For this review, take the finished solid that the model builds, in its own axes (mm). A direction names the side the tool comes from. Round coordinates to 2 decimals unless told otherwise and drop trailing zeros. Loops run counter-clockwise (first coordinate to the right, second up) from the corner with the lowest first, then second, coordinate; pieces in that order, holes last. Notation, with made-up numbers: M 56,70 L 103,70 A30 ccw 103,102 Z; hole C 65.25,-30 d6. An arc over 180 degrees is marked long. One line per question, with ' | ' between items. Start each with the question number.
1) We need section A-A (x = -64). Give the boundary of the cut face in (y, z), and give its area (3 significant figures).
2) We need section D-D (z = 4.5). Give the boundary of the cut face in (x, y), and give its area (3 significant figures).
3) We need section B-B (z = 48). Give the boundary of the cut face in (x, y), and give its area (3 significant figures).
4) We need section C-C (y = 21). Give the boundary of the cut face in (x, z).
5) For pin 1 Ø12 at (x, y) = (-50.5, 51.5) entering from +Z; pin 2 Ø9 at (x, y) = (72.5, 54.5) entering from -Z; pin 3 Ø10 at (x, z) = (69, 23) entering from -Y; pin 4 Ø11 at (y, z) = (-12, 52.5) entering from +X, all flat-tipped, find the tip position at first contact; note any pin that passes through.
6) For probe 1 along X at (y, z) = (66.5, 5); probe 2 along Z at (x, y) = (64, 56); probe 3 along Y at (x, z) = (-70.5, 34), list the stretches that pass through material, from the lowest coordinate up. Write a range as from..to.
7) For faces 1 (the face through (5, -10, 50)), 2 (the face through (70, 57, 52.5)), 3 (the face through (-60, 40, 27)), 4 (the face through (-70, 62.5, 27)), 5 (the face through (0, -10, 45)), list the 3-axis set-ups (+Z, -Z, +X, -X, +Y, -Y) from which the entire face can be reached by the end or side of a thin tool; tool diameter is ignored.
8) Mouldability with a two-part tool opening along X and no side actions: class faces 6 (the face through (60, 32, 27)), 7 (the face through (-5, -10, 50)), 8 (the face through (1, -5, 27)) as pulls with the +X half, pulls with the -X half, needs draft (parallel to the pull), parting line crosses it, or undercut.
Autodesk Inventor part; units mm, degrees
ref_plane "YZ Plane" through (0, 0, 0) normal (1, 0, 0) x (0, 1, 0)
ref_plane "XZ Plane" through (0, 0, 0) normal (0, 1, 0) x (-1, 0, 0)
ref_plane "XY Plane" through (0, 0, 0) normal (0, 0, 1) x (1, 0, 0)
sketch "Boceto1" plane through (0, 0, 0) normal (0, 0, 1) x (1, 0, 0)
  line L0 (-80, 5) -> (80, 5)
  line L1 (80, 5) -> (80, -5)
  line L2 (80, -5) -> (-80, -5)
  line L3 (-80, -5) -> (-80, 5)
  line L4 (-80, 5) -> (80, -5) construction
  line L5 (80, 5) -> (-80, -5) construction
  point P0 (0, 0)
  dimension "d0" = 160
  dimension "d1" = 10
extrude "Extrusión1" add sketch "Boceto1" along normal blind 55
sketch "Boceto2" plane through (-80, 5, 0) normal (0, 1, 0) x (1, 0, 0)
  line L0 (0, 0) -> (0, -55)
  line L1 (0, -55) -> (160, -55)
  line L2 (0, 0) -> (20, 0)
  line L3 (20, 0) -> (20, -55)
  line L4 (20, -55) -> (0, -55)
  line L5 (0, -55) -> (0, 0)
  line L6 (160, 0) -> (160, -55)
  line L7 (160, 0) -> (140, 0)
  line L8 (140, 0) -> (140, -55)
  line L9 (140, -55) -> (160, -55)
  line L10 (160, -55) -> (160, 0)
  point P0 (80, 0)
  dimension "d4" = 20
  dimension "d5" = 20
extrude "Extrusión2" add sketch "Boceto2" along normal blind 70
sketch "Boceto3" plane through (-80, -5, 0) normal (-1, 0, 0) x (0, 0, 1)
  line L0 (0, 80) -> (55, 80)
  line L1 (20.5, 67.5) -> (34.5, 67.5)
  line L2 (34.5, 67.5) -> (34.5, 53.5)
  line L3 (34.5, 53.5) -> (20.5, 53.5)
  line L4 (20.5, 53.5) -> (20.5, 67.5)
  line L5 (20.5, 67.5) -> (34.5, 53.5) construction
  line L6 (34.5, 67.5) -> (20.5, 53.5) construction
  line L7 (0, 0) -> (0, 80)
  point P0 (0, 5)
  point P1 (27.5, 60.5)
  dimension "d10" = 14
  dimension "d11" = 14
  dimension "d12" = 20.5
  dimension "d13" = 12.5
extrude "Extrusión3" cut sketch "Boceto3" against normal blind 70
sketch "Boceto4" plane through (-80, -5, 0) normal (0, -1, 0) x (1, 0, 0)
  line L0 (140, 55) -> (20, 55)
  line L1 (75, 45) -> (85, 45)
  line L2 (85, 45) -> (85, 55)
  line L3 (85, 55) -> (75, 55)
  line L4 (75, 55) -> (75, 45)
  line L5 (75, 45) -> (85, 55) construction
  line L6 (85, 45) -> (75, 55) construction
  point P0 (80, 0)
  dimension "d17" = 10
extrude "Extrusión4" add sketch "Boceto4" along normal blind 10
sketch "Boceto5" plane through (80, -5, 55) normal (1, 0, 0) x (0, 0, -1)
  line L0 (2.5, 71) -> (47.5, 71)
  line L1 (47.5, 71) -> (47.5, 53)
  line L2 (47.5, 53) -> (2.5, 53)
  line L3 (2.5, 53) -> (2.5, 71)
  line L4 (2.5, 71) -> (47.5, 53) construction
  line L5 (47.5, 71) -> (2.5, 53) construction
  line L6 (0, 80) -> (55, 80)
  line L7 (55, 0) -> (55, 80)
  point P0 (55, 5)
  point P1 (25, 62)
  dimension "d20" = 45
  dimension "d21" = 18
  dimension "d22" = 9
  dimension "d23" = 7.5
extrude "Extrusión5" cut sketch "Boceto5" against normal blind 30
properties part number "camera_support"
Answers below:
1) outline: M -5,0 L 75,0 L 75,55 L -5,55 Z; hole M 48.5,20.5 L 62.5,20.5 L 62.5,34.5 L 48.5,34.5 Z | area: 4,200 mm^2
2) outline: M -80,-5 L 80,-5 L 80,75 L 60,75 L 60,5 L -60,5 L -60,75 L -80,75 Z | area: 4,400 mm^2
3) outline: M -80,-5 L -5,-5 L -5,-15 L 5,-15 L 5,-5 L 80,-5 L 80,48 L 60,48 L 60,5 L -60,5 L -60,75 L -80,75 Z; M 60,66 L 80,66 L 80,75 L 60,75 Z | area: 4,140 mm^2
4) outline: M -80,0 L -60,0 L -60,55 L -80,55 Z; M 60,0 L 80,0 L 80,55 L 60,55 Z
5) pin 1: through | pin 2: z = 0 | pin 3: y = -5 | pin 4: x = 5
6) probe 1: -80..-60, 60..80 | probe 2: 0..7.5, 52.5..55 | probe 3: -5..48.5, 62.5..75
7) face 1: +Z, -Z, +X, -Y | face 2: +X | face 3: +Z, -Z, +Y | face 4: +X, -X | face 5: -Z, +X, -X, -Y
8) face 6: undercut | face 7: pulls with the -X half | face 8: needs draft
